from build123d import *

# Parameters (mm, degrees)
F0_W          = 25
F0_H          = 30
F1_DEPTH      = 4
F2_R          = 1.675
F3_DEPTH      = 25
F4_W          = 25
F4_H          = 11
F5_DEPTH      = 20
F7_DEPTH      = 6
F8_R          = 8
F9_DEPTH      = 6
F2_R_2        = 3
F10_DEPTH     = 2
F11_W         = 11
F11_H         = 24
F12_DEPTH     = 2
F13_R         = 5
F14_W         = 11
F14_H         = 24
F15_DEPTH     = 2
F16_DEPTH     = 2
F17_R         = 1.45
F18_DEPTH     = 25
F19_T1_DEPTH  = 49
F19_T6_DEPTH  = 49
F19_T11_DEPTH = 49
F19_T16_DEPTH = 49
F19_T21_DEPTH = 49
F20_DEPTH     = 25


# Not quite as in the source:
# - a fillet or chamfer that OpenCascade refuses, or shapes differently, is made with other operations: its cross-section is extruded or revolved along the edge and cut away or added


with BuildPart() as f1:
    # F0 (on Top) → F1 (new body)
    with BuildSketch(Plane.XY):
        with Locations((12.5, 15)):
            Rectangle(F0_W, F0_H)
    extrude(amount=F1_DEPTH)

    # F2 (on face) → F3 (cut)
    with BuildSketch(Plane.XY.offset(4)):
        with BuildLine():
            ThreePointArc((3.325, 18.5605346784), (5, 16.8855346784), (6.675, 18.5605346784))
            ThreePointArc((6.675, 18.5605346784), (5, 20.2355346784), (3.325, 18.5605346784))
        make_face()
        with Locations((20, 18.5605346784)):
            Circle(F2_R)
        with Locations((20, 3.5605346784)):
            Circle(F2_R)
        with Locations((5, 3.5605346784)):
            Circle(F2_R)
    extrude(amount=-F3_DEPTH, mode=Mode.SUBTRACT)

    # F4 (on face) → F5 (join)
    with BuildSketch(Plane.XY.offset(4)):
        with Locations((12.5, 24.5)):
            Rectangle(F4_W, F4_H)
    extrude(amount=F5_DEPTH)

    # F6 (on face) → F7 (cut)
    with BuildSketch(Plane(origin=(0, 30, 0), x_dir=(-1, 0, 0), z_dir=(0, 1, 0))):
        with BuildLine():
            ThreePointArc((-18.5, 24), (-12.5, 18), (-6.5, 24))
            Line((-6.5, 24), (-18.5, 24))
        make_face()
    extrude(amount=-F7_DEPTH, mode=Mode.SUBTRACT)

    # F8 (on face) → F9 (cut)
    with BuildSketch(Plane.XZ.offset(-19)):
        with Locations((12.5, 24)):
            Circle(F8_R)
    extrude(amount=-F9_DEPTH, mode=Mode.SUBTRACT)

    # F2 (on face) → F10 (cut)
    with BuildSketch(Plane.XY.offset(4)):
        with BuildLine():
            ThreePointArc((8, 18.5605346784), (5, 21.5605346784), (2, 18.5605346784))
            ThreePointArc((2, 18.5605346784), (5, 15.5605346784), (8, 18.5605346784))
        make_face()
        with BuildLine():
            ThreePointArc((3.325, 18.5605346784), (5, 20.2355346784), (6.675, 18.5605346784))
            ThreePointArc((6.675, 18.5605346784), (5, 16.8855346784), (3.325, 18.5605346784))
        make_face(mode=Mode.SUBTRACT)
        with Locations((20, 18.5605346784)):
            Circle(F2_R_2)
        with Locations((20, 18.5605346784)):
            Circle(F2_R, mode=Mode.SUBTRACT)
        with Locations((20, 3.5605346784)):
            Circle(F2_R_2)
        with Locations((20, 3.5605346784)):
            Circle(F2_R, mode=Mode.SUBTRACT)
        with Locations((5, 3.5605346784)):
            Circle(F2_R_2)
        with Locations((5, 3.5605346784)):
            Circle(F2_R, mode=Mode.SUBTRACT)
    extrude(amount=-F10_DEPTH, mode=Mode.SUBTRACT)

    # F11 (on face) → F12 (join)
    with BuildSketch(Plane(origin=(0, 0, 0), x_dir=(0, -1, 0), z_dir=(-1, 0, 0))):
        with Locations((-24.5, 12)):
            Rectangle(F11_W, F11_H)
    extrude(amount=F12_DEPTH)

    # F13
    f13_edges = [f1.edges().sort_by_distance(p)[0] for p in [
        (0, 0, 2),
        (25, 0, 2),
    ]]
    fillet(f13_edges, radius=F13_R)

    # F14 (on face) → F15 (join)
    with BuildSketch(Plane.YZ.offset(25)):
        with Locations((24.5, 12)):
            Rectangle(F14_W, F14_H)
    extrude(amount=F15_DEPTH)

    # F14 (on face) → F16 (join)
    with BuildSketch(Plane.YZ.offset(25)):
        with Locations((24.5, 12)):
            Rectangle(F14_W, F14_H)
    extrude(amount=F16_DEPTH)

    # F17 (on face) → F18 (cut)
    with BuildSketch(Plane.XY.offset(24)):
        with Locations((0.45, 25.55)):
            Circle(F17_R)
        with Locations((24.55, 25.55)):
            Circle(F17_R)
    extrude(amount=-F18_DEPTH, mode=Mode.SUBTRACT)

    # F19: fillet of radius 5 on 4 edges, made by hand

    # F19_s2 → F19_t1 (cut)
    with BuildSketch(Plane.XY.offset(-12.5)):
        with BuildLine():
            ThreePointArc((-2, 25), (-0.5355339059, 28.5355339059), (3, 30))
            Line((3, 30), (-2, 30))
            Line((-2, 30), (-2, 25))
        make_face()
        with BuildLine():
            ThreePointArc((22, 30), (25.5355339059, 28.5355339059), (27, 25))
            Line((27, 25), (27, 30))
            Line((27, 30), (22, 30))
        make_face()
    extrude(amount=F19_T1_DEPTH, mode=Mode.SUBTRACT)


with BuildPart() as f19_tool4:
    # F19_s5 → F19_t6 (new body)
    with BuildSketch(Plane.XY.offset(-12.5)):
        with BuildLine():
            ThreePointArc((3, 19), (-0.5355339059, 20.4644660941), (-2, 24))
            Line((-2, 24), (-2, 19))
            Line((-2, 19), (3, 19))
        make_face()
    extrude(amount=F19_T6_DEPTH)

    split(bisect_by=Plane.YZ, keep=Keep.BOTTOM)


with BuildPart() as f1_1:
    add(f1.part)

    # F19_t3: cut F19_tool4
    add(f19_tool4.part, mode=Mode.SUBTRACT)


with BuildPart() as f19_tool9:
    # F19_s10 → F19_t11 (new body)
    with BuildSketch(Plane.XY.offset(-12.5)):
        with BuildLine():
            ThreePointArc((3, 19), (-0.5355339059, 20.4644660941), (-2, 24))
            Line((-2, 24), (-2, 19))
            Line((-2, 19), (3, 19))
        make_face()
    extrude(amount=F19_T11_DEPTH)

    split(bisect_by=Plane.XY.offset(4), keep=Keep.TOP)


with BuildPart() as f1_2:
    add(f1_1.part)

    # F19_t8: cut F19_tool9
    add(f19_tool9.part, mode=Mode.SUBTRACT)


with BuildPart() as f19_tool14:
    # F19_s15 → F19_t16 (new body)
    with BuildSketch(Plane.XY.offset(36.5)):
        with BuildLine():
            ThreePointArc((22, 19), (25.5355339059, 20.4644660941), (27, 24))
            Line((27, 24), (27, 19))
            Line((27, 19), (22, 19))
        make_face()
    extrude(amount=-F19_T16_DEPTH)

    split(bisect_by=Plane.XY.offset(4), keep=Keep.TOP)


with BuildPart() as f1_3:
    add(f1_2.part)

    # F19_t13: cut F19_tool14
    add(f19_tool14.part, mode=Mode.SUBTRACT)


with BuildPart() as f19_tool19:
    # F19_s20 → F19_t21 (new body)
    with BuildSketch(Plane.XY.offset(36.5)):
        with BuildLine():
            ThreePointArc((22, 19), (25.5355339059, 20.4644660941), (27, 24))
            Line((27, 24), (27, 19))
            Line((27, 19), (22, 19))
        make_face()
    extrude(amount=-F19_T21_DEPTH)

    split(bisect_by=Plane.YZ.offset(25), keep=Keep.TOP)


with BuildPart() as f1_4:
    add(f1_3.part)

    # F19_t18: cut F19_tool19
    add(f19_tool19.part, mode=Mode.SUBTRACT)

    # F2 (on face) → F20 (cut)
    with BuildSketch(Plane.XY.offset(4)):
        with BuildLine():
            ThreePointArc((8, 18.5605346784), (5, 21.5605346784), (2, 18.5605346784))
            ThreePointArc((2, 18.5605346784), (5, 15.5605346784), (8, 18.5605346784))
        make_face()
        with BuildLine():
            ThreePointArc((3.325, 18.5605346784), (5, 20.2355346784), (6.675, 18.5605346784))
            ThreePointArc((6.675, 18.5605346784), (5, 16.8855346784), (3.325, 18.5605346784))
        make_face(mode=Mode.SUBTRACT)
        with Locations((20, 18.5605346784)):
            Circle(F2_R_2)
        with Locations((20, 18.5605346784)):
            Circle(F2_R, mode=Mode.SUBTRACT)
        with BuildLine():
            ThreePointArc((3.325, 18.5605346784), (5, 16.8855346784), (6.675, 18.5605346784))
            ThreePointArc((6.675, 18.5605346784), (5, 20.2355346784), (3.325, 18.5605346784))
        make_face()
        with Locations((20, 18.5605346784)):
            Circle(F2_R)
    extrude(amount=F20_DEPTH, mode=Mode.SUBTRACT)


solid = f1_4.part
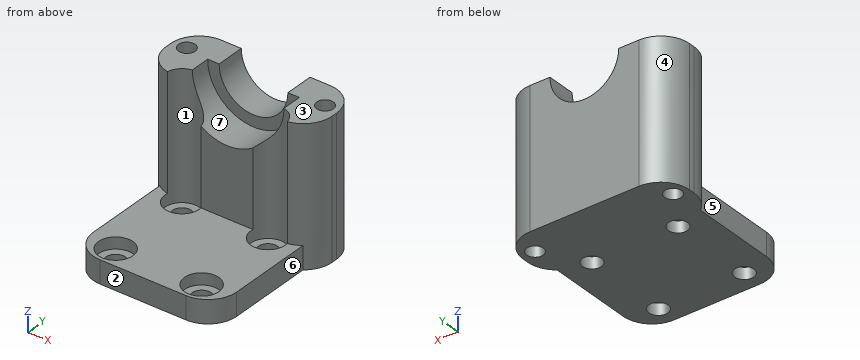
Geometry check sheet. Reference: the model listing, model coordinates, mm. Face numbers are marked on the shaded views. A direction names the side the tool comes from. Give positions to 0.01 mm unless a question says otherwise; leave off trailing zeros. Write each loop counter-clockwise with the first axis right and the second up, starting at its lowest first coordinate (ties: lowest second). Pieces come first, ordered by that corner, then holes.
1) Cross-section at D-D (x = 4). Record the boundary of the cut face in (y, z), plus the area to 3 significant figures.
Values follow:
outline: (0.1, 0) - (2.22, 0) - (2.22, 2) - (0.73, 2) - (0.73, 4) - (0.1, 4) - close; (4.9, 0) - (17.22, 0) - (17.22, 2) - (15.73, 2) - (15.73, 4) - (6.39, 4) - (6.39, 2) - (4.9, 2) - close; (19.9, 0) - (30, 0) - (30, 24) - (21.39, 24) - (21.39, 2) - (19.9, 2) - close
area: 258 mm2
2) Go/stop test with flat-tipped pins: pin 1 Ø2 at (x, y) = (5, 3.56) entering from -Z; pin 2 Ø5 at (y, z) = (19, 5.5) entering from -X; pin 3 Ø1.2 at (y, z) = (9.5, 2.5) entering from +X; pin 4 Ø1.5 at (x, z) = (8.5, 8) entering from -Y. Record where each tip stops, or that it passes through.
Values follow:
pin 1: passes through
pin 2: stops at x = -1.33
pin 3: stops at x = 25
pin 4: stops at y = 19
3) Cross-section at B-B (x = 1). Record the boundary of the cut face in (y, z), plus the area to 3 significant figures.
Values follow:
outline: (2, 0) - (24.21, 0) - (24.21, 24) - (19.42, 24) - (19.42, 4) - (2, 4) - close; (26.89, 0) - (29.58, 0) - (29.58, 24) - (26.89, 24) - close
area: 249 mm2
4) Set-up check for the marked faces 5, 6 and 7: record each of +Z, -Z, +X, -X, +Y, -Y from which the full face is reachable in a straight line by a thin tool's end or side.
Values follow:
face 5: +Z, -Z, -X, -Y
face 6: +Z, -Z, +X, -Y
face 7: +Z, -Y
5) Cross-section at A-A (z = 5). Record the boundary of the cut face in (x, y), plus the area to 3 significant figures.
Values follow:
outline: (-2, 24) arc R5 ccw to (2.05, 19.09) arc R3 cw to (7.97, 19) - (17.03, 19) arc R3 cw to (22.95, 19.09) arc R5 ccw to (27, 24) - (27, 25) arc R5 ccw to (22, 30) - (3, 30) arc R5 ccw to (-2, 25) - close; hole circle Ø2.9 at (0.45, 25.55); hole circle Ø2.9 at (24.55, 25.55)
area: 261 mm2
6) Cross-section at C-C (y = 25.55). Record the boundary of the cut face in (x, z).
Values follow:
outline: (-1.97, 0) - (-1, 0) - (-1, 24) - (-1.97, 24) - close; (1.9, 0) - (23.1, 0) - (23.1, 24) - (18.5, 24) arc R6 cw to (6.5, 24) - (1.9, 24) - close; (26, 0) - (26.97, 0) - (26.97, 24) - (26, 24) - close
7) Release check for a two-part mould opening along Y. For the marked faces 1, 2, 3 and 4 record: released by +Y, released by -Y, zero draft, split by the parting line, or undercut.
Values follow:
face 1: undercut
face 2: released by -Y
face 3: zero draft
face 4: released by +Y
8) Thickness scan on line 1 (Y direction, x = 5, z = 1.35); line 2 (X direction, y = 24.25, z = 1.5); line 3 (Y direction, x = 19.5, z = 3.25). Record the ranges inside material, lowest first.
Values follow:
line 1: y = 0 to 1.89, 5.24 to 16.89, 20.24 to 30
line 2: x = -2 to -0.19, 1.09 to 23.91, 25.19 to 27
line 3: y = 0 to 0.6, 6.52 to 15.6, 21.52 to 30
